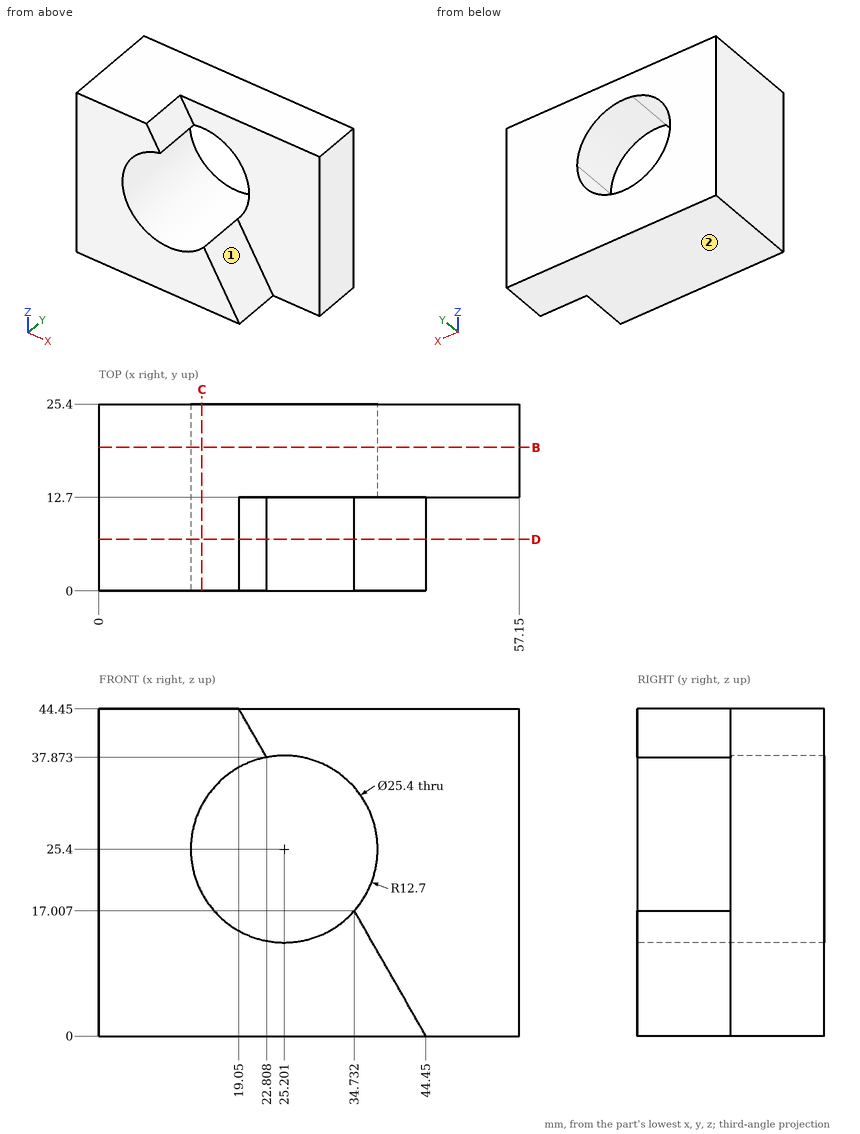
Study the drawing (mm; zero at the part's minimum x, y, z) and answer. A direction names the side the tool comes from. Coordinates: 2 decimals unless noted, no trailing zeros. Write each loop counter-clockwise with the first axis right and the second up, starting at its lowest first coordinate (ties: lowest second). Pieces come first, ordered by that corner, then holes. Notation, with made-up numbers: M 27.25,57 L 46.25,57 A20 cw 46.25,69 Z; hole C 16,42.5 d7. An arc over 180 degrees is marked long. Use a Markdown table: item, result. Add a question column.
1. Given P1, Ø23, axis at x = 25.2, z = 25.4, coming from the +Y side; P2, Ø1, axis at y = 11.5, z = 23.5, coming from the +X side, each flat-ended and moving along its own axis, determine where each tip first touches the part or whether it passes through.
2. Which of the six approach directions +Z, -Z, +X, -X, +Y, -Y give full straight-line access (tool end or side, diameter ignored) to the marked faces 1 and 2?
3. Section B-B (y = 19.5) is taken. Give the vertices of the cut face in (x, z).
4. Section C-C (x = 14) is taken. Give the vertices of the cut face in (y, z), plus the area to 3 significant figures.
5. Straight lines are drawn through the part: line 1 along X through (y, z) = (18, 25.4); line 2 along X through (y, z) = (8.25, 25.4); line 3 along Y through (x, z) = (44.5, 26). For each, find the intervals that lie inside material, in ascending order. Write a range as [from, to].
6. Section D-D (y = 7) is taken. Give the vertices of the cut face in (x, z).
Data:
| question | item | result |
|---|---|---|
| 1 | P1 | passes through |
| 1 | P2 | stops at x = 12.73 |
| 2 | face 1 | +Z, +X, -Y |
| 2 | face 2 | -Z, +X, -X, +Y, -Y |
| 3 | outline | M 0,0 L 57.15,0 L 57.15,44.45 L 0,44.45 Z; hole M 22.81,37.87 A12.7 ccw long 34.73,17.01 A12.7 ccw 37.9,25.4 A12.7 ccw Z |
| 4 | outline | M 0,0 L 25.4,0 L 25.4,19.41 L 0,19.41 Z; M 0,31.39 L 25.4,31.39 L 25.4,44.45 L 0,44.45 Z |
| 4 | area | 825 mm2 |
| 5 | line 1 | x = [0, 12.5], [37.9, 57.15] |
| 5 | line 2 | x = [0, 12.5] |
| 5 | line 3 | y = [12.7, 25.4] |
| 6 | outline | M 0,0 L 44.45,0 L 34.73,17.01 A12.7 cw long 22.81,37.87 L 19.05,44.45 L 0,44.45 Z |
